```python
from build123d import *

# Parameters (mm, degrees)
SKETCH1_W                = 38.1
SKETCH1_H                = 38.1
SKETCH1_W_2              = 31.75
SKETCH1_H_2              = 31.75
BOSS_EXTRUDE1_DEPTH      = 279.4
X_0_397_DIAMETER_HOLE1_D = 10.0838


with BuildPart() as part:
    # Sketch1 → Boss-Extrude1 (new body)
    with BuildSketch(Plane(origin=(0, 0, 0), x_dir=(1, 0, 0), z_dir=(0, 1, 0))):
        with Locations((19.05, 19.05)):
            Rectangle(SKETCH1_W, SKETCH1_H)
        with Locations((19.05, 19.05)):
            Rectangle(SKETCH1_W_2, SKETCH1_H_2, mode=Mode.SUBTRACT)
    extrude(amount=BOSS_EXTRUDE1_DEPTH)

    # X (0.397) Diameter Hole1 (through all)
    with Locations(Plane.XY):
        with Locations((19.05, 260.35), (19.05, 19.05)):
            Hole(X_0_397_DIAMETER_HOLE1_D / 2)


solid = part.part
```
CAD build for the part. Positions are in the model's coordinates, mm. A direction names the side the tool comes from. Coordinates: 2 decimals unless noted, no trailing zeros. Write each loop counter-clockwise with the first axis right and the second up, starting at its lowest first coordinate (ties: lowest second). Pieces come first, ordered by that corner, then holes. Notation, with made-up numbers: (29, 18) -> (67, 18) arc R14 cw to (67, 45) -> close; hole circle Ø1 at (-34.75, 41). An arc over 180 degrees is marked (long way). Use CSV: the item, a comma, the result in double quotes. Start each with the question number.
Item 1: Tool access for faces 5 (the flat face through (36, 279.4, -19)), 6 (the flat face through (34.925, 138, -19)): list every direction of +Z, -Z, +X, -X, +Y, -Y with a clear straight run to the whole face (end or side of a thin tool).
Item 2: Band-saw the part on A-A, the plane x = 19.05. Write the cut outline in (y, z) (3 decimals).
Item 3: Band-saw the part on B-B, the plane z = -28. Write the cut outline in (x, y) (3 decimals).
Item 4: Drop flat-ended pins along their axis: P1, Ø4, axis at y = 244.5, z = -9.5, coming from the -X side; P2, Ø9, axis at x = 19.05, y = 260.35, coming from the +Z side. Give the stop position or say it passes through.
Item 5: Band-saw the part on C-C, the plane y = 238. Write the cut outline in (x, z) (3 decimals), plus the area to 3 significant figures.
Item 6: Two-plate mould, pull along X, no slides. Class faces 1 (the flat face through (19, 138, -38.1)), 2 (the flat face through (0, 138, -19)), 3 (the cylindrical face through (19.71, 265.35, -1.61)), 4 (the cylindrical face through (16.34, 23.3, -1.61)): +X half, -X half, draft (parallel to the pull), parting line (faces both ways), or undercut.
Item 7: Wall check: probe 1 along Y at (x, z) = (19, -1); probe 2 along Z at (x, y) = (18, 11) (3 decimals); probe 3 along X at (y, z) = (28, -26) (3 decimals). Give the ranges that are in metal, low to high.
Response values:
1,face 5,"+Z, -Z, +X, -X, +Y"
1,face 6,"+Y, -Y"
2,outline,"(0, -38.1) -> (14.008, -38.1) -> (14.008, -34.925) -> (0, -34.925) -> close; (0, -3.175) -> (14.008, -3.175) -> (14.008, 0) -> (0, 0) -> close; (24.092, -38.1) -> (255.308, -38.1) -> (255.308, -34.925) -> (24.092, -34.925) -> close; (24.092, -3.175) -> (255.308, -3.175) -> (255.308, 0) -> (24.092, 0) -> close; (265.392, -38.1) -> (279.4, -38.1) -> (279.4, -34.925) -> (265.392, -34.925) -> close; (265.392, -3.175) -> (279.4, -3.175) -> (279.4, 0) -> (265.392, 0) -> close"
3,outline,"(0, 0) -> (3.175, 0) -> (3.175, 279.4) -> (0, 279.4) -> close; (34.925, 0) -> (38.1, 0) -> (38.1, 279.4) -> (34.925, 279.4) -> close"
4,P1,"stops at x = 0"
4,P2,"passes through"
5,outline,"(0, -38.1) -> (38.1, -38.1) -> (38.1, 0) -> (0, 0) -> close; hole (3.175, -34.925) -> (34.925, -34.925) -> (34.925, -3.175) -> (3.175, -3.175) -> close"
5,area,"444 mm2"
6,face 1,"draft"
6,face 2,"-X half"
6,face 3,"undercut"
6,face 4,"undercut"
7,probe 1,"y = 0 to 14.01, 24.09 to 255.31, 265.39 to 279.4"
7,probe 2,"z = -38.1 to -34.925, -3.175 to 0"
7,probe 3,"x = 0 to 3.175, 34.925 to 38.1"
